Solid Edge part; units mm, degrees
sketch "Sketch1" plane through (0, 0, 0) normal (0, 0, 1) x (1, 0, 0)
  line L0 (-250, -250) -> (250, -250)
  line L1 (250, -250) -> (250, 250)
  line L2 (250, 250) -> (-250, 250)
  line L3 (-250, 250) -> (-250, -250)
  line L4 (-241, -241) -> (241, -241)
  line L5 (241, -241) -> (241, 241)
  line L6 (241, 241) -> (-241, 241)
  line L7 (-241, 241) -> (-241, -241)
extrude "Protrusion1" add sketch "Sketch1" along normal blind 100
sketch "Sketch2" plane through (0, 0, 100) normal (0, 0, 1) x (1, 0, 0)
  line L0 (0, 250) -> (-50, 250)
  line L1 (-50, 250) -> (-50, 241)
  line L2 (-50, 241) -> (0, 241)
  line L3 (50, 241) -> (0, 241)
  line L4 (50, 250) -> (50, 241)
  line L5 (0, 250) -> (50, 250)
  line L6 (-50, -250) -> (50, -250)
  line L7 (50, -250) -> (50, -241)
  line L8 (50, -241) -> (-50, -241)
  line L9 (-50, -241) -> (-50, -250)
extrude "ExtrudedProtrusion_2" add sketch "Sketch2" along normal blind 200
hole "Hole_1" at (250, -125, 50) direction (-1, 0, 0) diameter 10 end up to next
hole "Hole_2" at (250, 125, 50) direction (-1, 0, 0) diameter 10 end up to next
hole "Hole_Screw1" at (250, 0, 50) direction (-1, 0, 0) diameter 15 end up to next
hole "Hole_4" at (-250, 125, 50) direction (1, 0, 0) diameter 10 end up to next
hole "Hole1" at (-250, -125, 50) direction (1, 0, 0) diameter 10 end up to next
hole "Hole_Screw2" at (-250, 0, 50) direction (1, 0, 0) diameter 15 end up to next
hole "Hole_7" at (25, -250, 250) direction (0, 1, 0) diameter 10 end up to next
hole "Hole2" at (0, -250, 200) direction (0, 1, 0) diameter 10 end up to next
hole "Hole_9" at (25, 250, 250) direction (0, -1, 0) diameter 10 end up to next
hole "Hole3" at (0, 250, 200) direction (0, -1, 0) diameter 10 end up to next
fillet "Round1" radius 10 4 edges at (-50, 245.5, 300) (50, 245.5, 300) (-50, -245.5, 300) (50, -245.5, 300)
Geometry check sheet. Reference: the model listing, model coordinates, mm. A direction names the side the tool comes from. Give positions to 0.01 mm unless a question says otherwise; leave off trailing zeros. Order: outer loops, then holes, each group sorted by start corner. A loop starts at its lowest first (then second) coordinate and runs counter-clockwise, first axis right, second up. Notation, with made-up numbers: (9, 3) -> (31, 3) arc R18 cw to (31, 21) -> close; hole circle Ø10 at (81.5, 27). An arc over 180 degrees is marked (long way). Write each question's results on one line, items separated by ' | '. Start each with the question number.
(1) Mould release check, pull along X, two halves, no side actions. Record for faces 5 (the face through (-245.563, 2.253, 57.154)), 6 (the face through (3, 241, 81)), 7 (the face through (250, -3, 38)): pulls with the +X half, pulls with the -X half, needs draft (parallel to the pull), parting line crosses it, or undercut.
(2) Gauge pin test, flat ends, axial feed: P1, Ø7, axis at y = 247, z = 194.5, coming from the +X side; P2, Ø9, axis at y = 125, z = 50, coming from the +X side; P3, Ø10, axis at y = -247, z = 167, coming from the -X side. Record the tip position at first contact, or that the pin passes through.
(3) Scan lines: line 1 (Z direction, x = 0, y = -245.75); line 2 (Y direction, x = 243, z = 50); line 3 (Z direction, x = -243.5, y = -125). Record each from-to range of solid material in increasing order.
(4) Sectioned sample at C-C (y = 0). Enter the section's corners in (x, z), plus the area to 3 significant figures.
(5) Sectioned sample at A-A (y = -170.5). Enter the section's corners in (x, z).
(6) Access from +Z, -Z, +X, -X, +Y, -Y to the whole of each face (thin tool, end or side, straight path). Record for faces 1 (the face through (246, 112, 100)), 2 (the face through (-3, -250, 81)), 3 (the face through (-3, -241, 81)), 4 (the face through (-247, 112, 100)).
(7) Sectioned sample at D-D (z = 32.5). Enter the section's corners in (x, y).
Answer below:
1) face 5: needs draft | face 6: undercut | face 7: pulls with the +X half
2) P1: x = 50 | P2: through | P3: x = -50
3) line 1: 0 to 195, 205 to 300 | line 2: -250 to -130, -120 to -7.5, 7.5 to 120, 130 to 250 | line 3: 0 to 45, 55 to 100
4) outline: (-250, 0) -> (-241, 0) -> (-241, 42.5) -> (-250, 42.5) -> close; (-250, 57.5) -> (-241, 57.5) -> (-241, 100) -> (-250, 100) -> close; (241, 0) -> (250, 0) -> (250, 42.5) -> (241, 42.5) -> close; (241, 57.5) -> (250, 57.5) -> (250, 100) -> (241, 100) -> close | area: 1,530 mm2
5) outline: (-250, 0) -> (-241, 0) -> (-241, 100) -> (-250, 100) -> close; (241, 0) -> (250, 0) -> (250, 100) -> (241, 100) -> close
6) face 1: +Z, +X, +Y, -Y | face 2: +Z, -Z, +X, -X, -Y | face 3: +Z, -Z | face 4: +Z, -X, +Y, -Y
7) outline: (-250, -250) -> (250, -250) -> (250, 250) -> (-250, 250) -> close; hole (-241, -241) -> (241, -241) -> (241, 241) -> (-241, 241) -> close
